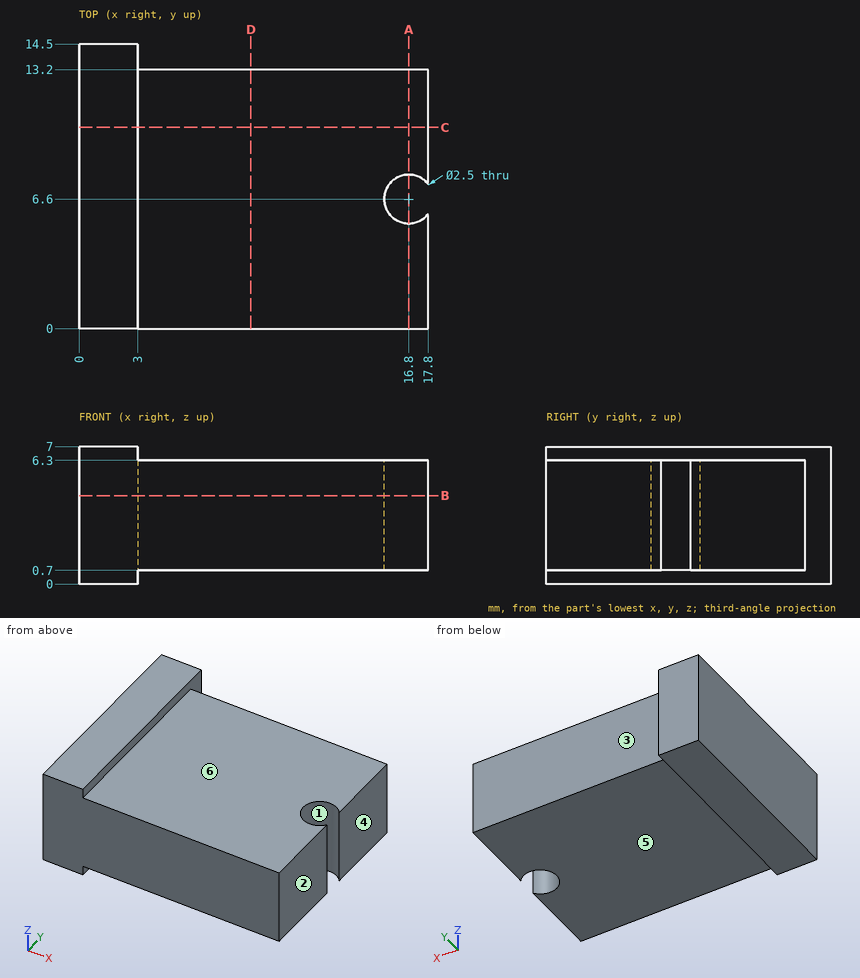
Source: three-view drawing plus pictorial views. Frame: mm from the lowest corner of the part. A direction names the side the tool comes from. Round coordinates to 2 decimals unless told otherwise and drop trailing zeros. Loops run counter-clockwise (first coordinate to the right, second up) from the corner with the lowest first, then second, coordinate; pieces in that order, holes last.
Q1. Section B-B, the plane z = 4.5. Return loops of the section in (x, y).
Q2. Section A-A, the plane x = 16.8. Return loops of the section in (y, z), plus the area to 3 significant figures.
Q3. Section C-C, the plane y = 10.25. Return loops of the section in (x, z).
Q4. Access query for the marked faces 4, 5 and 6. Directions: +Z, -Z, +X, -X, +Y, -Y. A direction counts if a zero-diameter tool reaches every point of the face in a straight line with its end or side. Return the directions, or none.
Q5. Section D-D, the plane x = 8.75. Return loops of the section in (y, z).
Q6. Mould query, pull axis Y, two halves, no side actions, for the marked faces 1, 2 and 3. Classes: pulls with the +Y half, pulls with the -Y half, needs draft (parallel to the pull), parting line crosses it, or undercut.
Q7. First-contact query: P1, Ø6.5, axis at x = 12, y = 9.5, coming from the -Z side; P2, Ø6, axis at x = 16, y = 4, coming from the +Z side; P3, Ø1.7, axis at x = 9, z = 2.5, coming from the +Y side. Flat tips, straight axial feed; report the tip coordinate or a pass-through.
Q8. Ray query, line 1 (Y direction, x = 16.8, z = 3.4); line 2 (Z direction, x = 10.5, y = 11.5); line 3 (X direction, y = 6.6, z = 3.65). Return the intervals inside material, ascending.
Solutions:
1. outline: (0, 0) - (17.8, 0) - (17.8, 5.85) arc R1.25 cw (long way) to (17.8, 7.35) - (17.8, 13.2) - (3, 13.2) - (3, 14.5) - (0, 14.5) - close
2. outline: (0, 0.7) - (5.35, 0.7) - (5.35, 6.3) - (0, 6.3) - close; (7.85, 0.7) - (13.2, 0.7) - (13.2, 6.3) - (7.85, 6.3) - close
2. area: 59.9 mm2
3. outline: (0, 0) - (3, 0) - (3, 0.7) - (17.8, 0.7) - (17.8, 6.3) - (3, 6.3) - (3, 7) - (0, 7) - close
4. face 4: +Z, -Z, +X, +Y, -Y
4. face 5: -Z, +X, +Y, -Y
4. face 6: +Z, +X, +Y, -Y
5. outline: (0, 0.7) - (13.2, 0.7) - (13.2, 6.3) - (0, 6.3) - close
6. face 1: undercut
6. face 2: needs draft
6. face 3: pulls with the +Y half
7. P1: stops at z = 0.7
7. P2: stops at z = 6.3
7. P3: stops at y = 13.2
8. line 1: y = 0 to 5.35, 7.85 to 13.2
8. line 2: z = 0.7 to 6.3
8. line 3: x = 0 to 15.55
